The listing builds one solid part. Answer for the finished solid, in the listing's coordinates (mm). Round coordinates to 2 decimals unless told otherwise and drop trailing zeros. Write each loop counter-clockwise with the first axis right and the second up, starting at its lowest first coordinate (ties: lowest second). Pieces come first, ordered by that corner, then holes. Notation, with made-up numbers: (-1, 26) - (16, 26) arc R18 cw to (16, 43) - close; hole circle Ø6 at (58, 41.5). An arc over 180 degrees is marked (long way). Return JSON: item names as keys, results as strings. Group by question number.
(1) Section B-B, the plane y = 43.5 is taken. Write down the section's boundary in (x, z).
(2) Find the intervals of material crossed by line 1 along Y through (x, z) = (1.15, 6); line 2 along X through (y, z) = (45.5, 8.75); line 3 along X through (y, z) = (31.5, 4.75), in increasing order. Write a range as [from, to].
(3) Section A-A, the plane y = 10 is taken. Write down the section's boundary in (x, z), then the cut area to 3 significant figures.
(4) Section C-C, the plane x = 77 is taken. Give the number of separate pieces and of enclosed holes in the cut face, then the cut area to 3 significant figures.
```python
from build123d import *

# Parameters (mm, degrees)
ESQUISSE1_W             = 130
ESQUISSE1_H             = 65
BOSS_EXTRU_1_DEPTH      = 12
ESQUISSE2_R             = 1.6
ENL_V_MAT_EXTRU_1_DEPTH = 13
ENL_V_MAT_EXTRU_6_DEPTH = 10
D_GAGEMENT_M61_D        = 6.6
D_GAGEMENT_M61_DEPTH    = 6.017159957
D_GAGEMENT_M61_TIP      = 1.982840043
ESQUISSE10_R            = 4
ENL_V_MAT_EXTRU_7_DEPTH = 2
ENL_V_MAT_EXTRU_9_DEPTH = 1
ESQUISSE12_W            = 105
ESQUISSE12_H            = 1.5
ESQUISSE12_W_2          = 110
BOSS_EXTRU_2_DEPTH      = 10


with BuildPart() as part:
    # Esquisse1 → Boss.-Extru.1 (new body)
    with BuildSketch(Plane.XY):
        with Locations((65, 32.5)):
            Rectangle(ESQUISSE1_W, ESQUISSE1_H)
    extrude(amount=BOSS_EXTRU_1_DEPTH)

    # Esquisse2 → Enlèv. mat.-Extru.1 (cut, through all)
    with BuildSketch(Plane.XY.offset(12)):
        with Locations((5, 55)):
            Circle(ESQUISSE2_R)
        with Locations((29, 55)):
            Circle(ESQUISSE2_R)
        with Locations((53, 55)):
            Circle(ESQUISSE2_R)
        with Locations((77, 55)):
            Circle(ESQUISSE2_R)
        with Locations((101, 55)):
            Circle(ESQUISSE2_R)
        with Locations((125, 55)):
            Circle(ESQUISSE2_R)
        with Locations((5, 10)):
            Circle(ESQUISSE2_R)
        with Locations((29, 10)):
            Circle(ESQUISSE2_R)
        with Locations((53, 10)):
            Circle(ESQUISSE2_R)
        with Locations((77, 10)):
            Circle(ESQUISSE2_R)
        with Locations((101, 10)):
            Circle(ESQUISSE2_R)
        with Locations((125, 10)):
            Circle(ESQUISSE2_R)
        with Locations((90, 32.5)):
            Circle(ESQUISSE2_R)
        with Locations((40, 32.5)):
            Circle(ESQUISSE2_R)
    extrude(amount=-ENL_V_MAT_EXTRU_1_DEPTH, mode=Mode.SUBTRACT)

    # Esquisse6 → Enlèv. mat.-Extru.6 (cut)
    with BuildSketch(Plane.XY.offset(12)):
        with BuildLine():
            Line((8, 50), (122, 50))
            ThreePointArc((122, 50), (124.121320344, 49.121320344), (125, 47))
            Line((125, 47), (125, 18))
            ThreePointArc((125, 18), (124.121320344, 15.878679656), (122, 15))
            Line((122, 15), (8, 15))
            ThreePointArc((8, 15), (5.878679656, 15.878679656), (5, 18))
            Line((5, 18), (5, 25))
            ThreePointArc((5, 25), (5.878679656, 27.121320344), (8, 28))
            Line((8, 28), (109, 28))
            ThreePointArc((109, 28), (111.121320344, 28.878679656), (112, 31))
            Line((112, 31), (112, 34))
            ThreePointArc((112, 34), (111.121320344, 36.121320344), (109, 37))
            Line((109, 37), (8, 37))
            ThreePointArc((8, 37), (5.878679656, 37.878679656), (5, 40))
            Line((5, 40), (5, 47))
            ThreePointArc((5, 47), (5.878679656, 49.121320344), (8, 50))
        make_face()
    extrude(amount=-ENL_V_MAT_EXTRU_6_DEPTH, mode=Mode.SUBTRACT)

    # Dégagement M61
    with Locations(Plane.ZY):
        with Locations((6, 43.5), (6, 21.5)):
            Hole(D_GAGEMENT_M61_D / 2, depth=D_GAGEMENT_M61_DEPTH)
            with Locations((0, 0, -(D_GAGEMENT_M61_DEPTH + D_GAGEMENT_M61_TIP / 2))):  # 118° drill point
                Cone(0, D_GAGEMENT_M61_D / 2, D_GAGEMENT_M61_TIP, mode=Mode.SUBTRACT)

    # Esquisse10 → Enlèv. mat.-Extru.7 (cut)
    with BuildSketch(Plane.ZY):
        with Locations((6, 21.5)):
            Circle(ESQUISSE10_R)
        with Locations((6, 43.5)):
            Circle(ESQUISSE10_R)
    extrude(amount=-ENL_V_MAT_EXTRU_7_DEPTH, mode=Mode.SUBTRACT)

    # Esquisse11 → Enlèv. mat.-Extru.9 (cut)
    with BuildSketch(Plane.XY.offset(12)):
        with BuildLine():
            Line((125, 12.5), (5, 12.5))
            ThreePointArc((5, 12.5), (3.585786438, 13.085786438), (3, 14.5))
            Line((3, 14.5), (3, 28.315802411))
            ThreePointArc((3, 28.315802411), (3.585786438, 29.730015973), (5, 30.315802411))
            Line((5, 30.315802411), (108, 30.315802411))
            ThreePointArc((108, 30.315802411), (109.414213562, 30.901588849), (110, 32.315802411))
            Line((110, 32.315802411), (110, 33.034217912))
            ThreePointArc((110, 33.034217912), (109.414213562, 34.448431474), (108, 35.034217912))
            Line((108, 35.034217912), (5, 35.034217912))
            ThreePointArc((5, 35.034217912), (3.585786438, 35.620004349), (3, 37.034217912))
            Line((3, 37.034217912), (3, 50.5))
            ThreePointArc((3, 50.5), (3.585786438, 51.914213562), (5, 52.5))
            Line((5, 52.5), (125, 52.5))
            ThreePointArc((125, 52.5), (126.414213562, 51.914213562), (127, 50.5))
            Line((127, 50.5), (127, 14.5))
            ThreePointArc((127, 14.5), (126.414213562, 13.085786438), (125, 12.5))
        make_face()
        with BuildLine():
            Line((6, 51.5), (124, 51.5))
            ThreePointArc((124, 51.5), (125.414213562, 50.914213562), (126, 49.5))
            Line((126, 49.5), (126, 15.5))
            ThreePointArc((126, 15.5), (125.414213562, 14.085786438), (124, 13.5))
            Line((124, 13.5), (6, 13.5))
            ThreePointArc((6, 13.5), (4.585786438, 14.085786438), (4, 15.5))
            Line((4, 15.5), (4, 27.315802411))
            ThreePointArc((4, 27.315802411), (4.585786438, 28.730015973), (6, 29.315802411))
            Line((6, 29.315802411), (109, 29.315802411))
            ThreePointArc((109, 29.315802411), (110.414213562, 29.901588849), (111, 31.315802411))
            Line((111, 31.315802411), (111, 34.034217912))
            ThreePointArc((111, 34.034217912), (110.414213562, 35.448431474), (109, 36.034217912))
            Line((109, 36.034217912), (6, 36.034217912))
            ThreePointArc((6, 36.034217912), (4.585786438, 36.620004349), (4, 38.034217912))
            Line((4, 38.034217912), (4, 49.5))
            ThreePointArc((4, 49.5), (4.585786438, 50.914213562), (6, 51.5))
        make_face(mode=Mode.SUBTRACT)
    extrude(amount=-ENL_V_MAT_EXTRU_9_DEPTH, mode=Mode.SUBTRACT)

    # Esquisse12 → Boss.-Extru.2 (add)
    with BuildSketch(Plane.XY.offset(2)):
        with Locations((62.5, 41.25)):
            Rectangle(ESQUISSE12_W, ESQUISSE12_H)
        with Locations((65, 45.75)):
            Rectangle(ESQUISSE12_W_2, ESQUISSE12_H)
        with Locations((65, 19.25)):
            Rectangle(ESQUISSE12_W_2, ESQUISSE12_H)
        with Locations((62.5, 23.75)):
            Rectangle(ESQUISSE12_W, ESQUISSE12_H)
    extrude(amount=BOSS_EXTRU_2_DEPTH)


solid = part.part
```
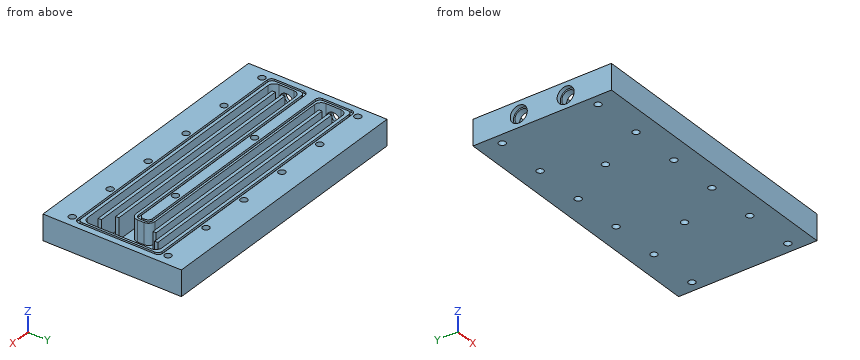
Working result:
{
 "1": {"outline": "(0, 0) - (130, 0) - (130, 12) - (127, 12) - (127, 11) - (126, 11) - (126, 12) - (125, 12) - (125, 2) - (5, 2) - (5, 2.7) - (2, 2.7) - (2, 2) - (0, 2) - close; (0, 10) - (2, 10) - (2, 9.3) - (5, 9.3) - (5, 12) - (4, 12) - (4, 11) - (3, 11) - (3, 12) - (0, 12) - close"},
 "2": {"line 1": "y = [0, 17.5], [25.5, 39.5], [47.5, 65]", "line 2": "x = [2, 5], [10, 120], [125, 130]", "line 3": "x = [0, 38.75], [41.25, 88.75], [91.25, 112], [125, 130]"},
 "3": {"outline": "(0, 0) - (3.4, 0) - (3.4, 12) - (0, 12) - close; (6.6, 0) - (27.4, 0) - (27.4, 12) - (6.6, 12) - close; (30.6, 0) - (51.4, 0) - (51.4, 12) - (30.6, 12) - close; (54.6, 0) - (75.4, 0) - (75.4, 12) - (54.6, 12) - close; (78.6, 0) - (99.4, 0) - (99.4, 12) - (78.6, 12) - close; (102.6, 0) - (123.4, 0) - (123.4, 12) - (102.6, 12) - close; (126.6, 0) - (130, 0) - (130, 12) - (126.6, 12) - close", "area": "1,330 mm^2"},
 "4": {"separate pieces": "3", "enclosed holes": "0", "area": "499 mm^2"}
}
